CAD build for the part. Positions are in the model's coordinates, mm. A direction names the side the tool comes from. Round coordinates to 2 decimals unless told otherwise and drop trailing zeros. Order: outer loops, then holes, each group sorted by start corner. A loop starts at its lowest first (then second) coordinate and runs counter-clockwise, first axis right, second up. Notation, with made-up numbers: M -20.5,-5 L 15.5,-5 A21 cw 15.5,28 Z; hole C 81.5,-40 d2. An arc over 180 degrees is marked long. Answer as a JSON object with one key per item and string values.
```python
from build123d import *

# Parameters (mm, degrees)
EXTRUDE_3_DEPTH     = 1.7
SKETCH_4_R          = 0.81
EXTRUDE_4_DEPTH     = 3.7
SKETCH_5_W          = 79
SKETCH_5_H          = 14.47
EXTRUDE_5_DEPTH     = 5
SKETCH_6_W          = 79
SKETCH_6_H          = 31.63
EXTRUDE_6_DEPTH     = 5
FILLET_1_R          = 0.31
FILLET_2_R          = 0.5
FILLET_3_R          = 0.5
FILLET_5_R          = 0.5
SKETCH_8_W          = 40
SKETCH_8_H          = 31.63
EXTRUDE_7_DEPTH     = 5
FILLET_6_R          = 0.5
SKETCH_9_R          = 0.975
CUT_EXTRUDE_1_DEPTH = 5
FILLET_7_R          = 0.5


with BuildPart() as part:
    # 草图1 → 凸台-拉伸3 (new body)
    with BuildSketch(Plane.XY):
        with BuildLine():
            Line((0, 1.75), (55.5, 1.75))
            ThreePointArc((55.5, 1.75), (57.25, 0), (55.5, -1.75))
            Line((55.5, -1.75), (0, -1.75))
            ThreePointArc((0, -1.75), (-1.75, 0), (0, 1.75))
        make_face()
    extrude(amount=EXTRUDE_3_DEPTH)

    # 草图4 → 凸台-拉伸4 (add)
    with BuildSketch(Plane(origin=(0, 0, 0), x_dir=(-1, 0, 0), z_dir=(0, 0, -1))):
        Circle(SKETCH_4_R)
        with Locations((-55.5, 0)):
            Circle(SKETCH_4_R)
    extrude(amount=-EXTRUDE_4_DEPTH)

    # 草图5 → 凸台-拉伸5 (add)
    with BuildSketch(Plane(origin=(0, 0, 0), x_dir=(-1, 0, 0), z_dir=(0, 0, -1))):
        with Locations((-27.5, -1.005)):
            Rectangle(SKETCH_5_W, SKETCH_5_H)
    extrude(amount=EXTRUDE_5_DEPTH)

    # 草图6 → 凸台-拉伸6 (add)
    with BuildSketch(Plane(origin=(0, 6.23, 0), x_dir=(1, 0, 0), z_dir=(0, 1, 0))):
        with Locations((27.5, -10.815)):
            Rectangle(SKETCH_6_W, SKETCH_6_H)
    extrude(amount=EXTRUDE_6_DEPTH)

    # 圆角1
    fillet_1_edges = [part.edges().sort_by_distance(p)[0] for p in [
        (27.5, 6.23, 0),
    ]]
    fillet(fillet_1_edges, radius=FILLET_1_R)

    # 圆角2
    fillet_2_edges = [part.edges().sort_by_distance(p)[0] for p in [
        (67, -8.24, -2.5),
    ]]
    fillet(fillet_2_edges, radius=FILLET_2_R)

    # 圆角3
    fillet_3_edges = [part.edges().sort_by_distance(p)[0] for p in [
        (-12, -8.24, -2.5),
    ]]
    fillet(fillet_3_edges, radius=FILLET_3_R)

    # 圆角5
    fillet_5_edges = [part.edges().sort_by_distance(p)[0] for p in [
        (67, 11.23, 10.815),
    ]]
    fillet(fillet_5_edges, radius=FILLET_5_R)

    # 草图8 → 凸台-拉伸7 (add)
    with BuildSketch(Plane(origin=(0, -8.24, 0), x_dir=(-1, 0, 0), z_dir=(0, -1, 0))):
        with Locations((-35.5, -10.815)):
            Rectangle(SKETCH_8_W, SKETCH_8_H)
    extrude(amount=EXTRUDE_7_DEPTH)

    # 圆角6
    fillet_6_edges = [part.edges().sort_by_distance(p)[0] for p in [
        (67, 8.48, 26.63),
        (66.853553391, 11.083553391, 26.63),
        (2, -8.24, -5),
        (-11.853553391, -8.093553391, -5),
        (27.25, 11.23, -5),
        (66.853553391, 11.083553391, -5),
        (61, -8.24, -5),
        (66.853553391, -8.093553391, -5),
        (27.5, 6.23, 26.63),
        (-12, 8.73, 26.63),
        (27.25, 11.23, 26.63),
        (-12, 11.23, 10.815),
        (15.5, -8.24, 13.315),
        (15.5, -10.74, 26.63),
        (35.5, -8.24, 26.63),
        (55.5, -8.24, 13.315),
        (55.5, -10.74, 26.63),
        (55.5, -13.24, 10.815),
        (35.5, -13.24, 26.63),
        (15.5, -13.24, 10.815),
        (15.5, -10.74, -5),
        (-12, 1.745, -5),
        (55.5, -10.74, -5),
        (35.5, -13.24, -5),
        (67, 1.495, -5),
    ]]
    fillet(fillet_6_edges, radius=FILLET_6_R)

    # 草图9 → 切除-拉伸1 (cut)
    with BuildSketch(Plane.XY.offset(26.63)):
        with Locations((23.5, -10.74)):
            Circle(SKETCH_9_R)
        with Locations((47.5, -10.74)):
            Circle(SKETCH_9_R)
        with Locations((8, 8.73)):
            Circle(SKETCH_9_R)
        with Locations((47, 8.73)):
            Circle(SKETCH_9_R)
    extrude(amount=-CUT_EXTRUDE_1_DEPTH, mode=Mode.SUBTRACT)

    # 圆角7
    # the kernel refuses this fillet: 0.5 mm, written as the material it takes off along each edge
    with BuildSketch(Plane(origin=(-11.5, 6.73, 26.13), x_dir=(-1, 0, 0), z_dir=(0, -1, 0))) as fillet_7_piece_1_section:
        Polygon((0, 0), (FILLET_7_R * 1.02, 0), (FILLET_7_R * 1.02, -FILLET_7_R * 1.02), (0, -FILLET_7_R * 1.02), align=None)
    fillet_7_piece_1 = extrude(amount=FILLET_7_R * 1.02, mode=Mode.PRIVATE)
    fillet_7_piece_1 = fillet_7_piece_1 - Plane(origin=(-11.5, 6.73, 26.13), x_dir=(0.7071067811865475, 0, -0.7071067811865475), z_dir=(0, -1, 0)) * Sphere(FILLET_7_R, mode=Mode.PRIVATE)
    add(fillet_7_piece_1, mode=Mode.SUBTRACT)
    with BuildSketch(Plane(origin=(66.5, 6.73, 26.13), x_dir=(0, -1, 0), z_dir=(1, 0, 0))) as fillet_7_piece_2_section:
        Polygon((0, 0), (FILLET_7_R * 1.02, 0), (FILLET_7_R * 1.02, -FILLET_7_R * 1.02), (0, -FILLET_7_R * 1.02), align=None)
    fillet_7_piece_2 = extrude(amount=FILLET_7_R * 1.02, mode=Mode.PRIVATE)
    fillet_7_piece_2 = fillet_7_piece_2 - Plane(origin=(66.5, 6.73, 26.13), x_dir=(0, 0.7071067811865475, -0.7071067811865475), z_dir=(1, 0, 0)) * Sphere(FILLET_7_R, mode=Mode.PRIVATE)
    add(fillet_7_piece_2, mode=Mode.SUBTRACT)
    with BuildSketch(Plane(origin=(-12, 5.92, 0), x_dir=(1, 0, 0), z_dir=(0, -1, 0))) as fillet_7_piece_3:
        with BuildLine():
            CenterArc((FILLET_7_R, -FILLET_7_R), FILLET_7_R, 90, 90)
            Line((0, -FILLET_7_R), (0, 0))
            Line((0, 0), (FILLET_7_R, 0))
        make_face()
    extrude(amount=13.66, mode=Mode.SUBTRACT)
    with BuildSketch(Plane(origin=(67, -7.74, 0), x_dir=(0, 0, -1), z_dir=(0, 1, 0))) as fillet_7_piece_4:
        with BuildLine():
            CenterArc((FILLET_7_R, FILLET_7_R), FILLET_7_R, 180, 90)
            Line((0, FILLET_7_R), (0, 0))
            Line((0, 0), (FILLET_7_R, 0))
        make_face()
    extrude(amount=13.66, mode=Mode.SUBTRACT)
    with BuildSketch(Plane(origin=(-12, 6.23, 26.13), x_dir=(1, 0, 0), z_dir=(0, 0, -1))) as fillet_7_piece_5:
        with BuildLine():
            CenterArc((FILLET_7_R, -FILLET_7_R), FILLET_7_R, 90, 90)
            Line((0, -FILLET_7_R), (0, 0))
            Line((0, 0), (FILLET_7_R, 0))
        make_face()
    extrude(amount=25.82, mode=Mode.SUBTRACT)
    with BuildSketch(Plane(origin=(-12, 5.92, 0.31), x_dir=(0, 0, -1), z_dir=(0, -1, 0))) as fillet_7_piece_6:
        with BuildLine():
            CenterArc((0.31 + FILLET_7_R, FILLET_7_R), FILLET_7_R, 180, 90)
            Line((0.31 + FILLET_7_R, 0), (0.31, 0))
            Line((0.31, 0), (0.31, FILLET_7_R))
        make_face()
    revolve(axis=Axis((-12, 5.92, 0.31), (1, 0, 0)), revolution_arc=90, mode=Mode.SUBTRACT)
    with BuildSketch(Plane(origin=(67, 5.92, 0.31), x_dir=(0, 0, -1), z_dir=(0, -1, 0))) as fillet_7_piece_7:
        with BuildLine():
            CenterArc((0.31 + FILLET_7_R, -FILLET_7_R), FILLET_7_R, 90, 90)
            Line((0.31, -FILLET_7_R), (0.31, 0))
            Line((0.31, 0), (0.31 + FILLET_7_R, 0))
        make_face()
    revolve(axis=Axis((67, 5.92, 0.31), (1, 0, 0)), revolution_arc=90, mode=Mode.SUBTRACT)
    with BuildSketch(Plane(origin=(55.5, -8.24, 0), x_dir=(0, 1, 0), z_dir=(1, 0, 0))) as fillet_7_piece_8:
        with BuildLine():
            CenterArc((FILLET_7_R, -FILLET_7_R), FILLET_7_R, 90, 90)
            Line((0, -FILLET_7_R), (0, 0))
            Line((0, 0), (FILLET_7_R, 0))
        make_face()
    extrude(amount=11, mode=Mode.SUBTRACT)
    with BuildSketch(Plane(origin=(66.5, -7.74, 0), x_dir=(1, 0, 0), z_dir=(0, 1, 0))) as fillet_7_piece_9:
        with BuildLine():
            CenterArc((0.5 - FILLET_7_R, FILLET_7_R), FILLET_7_R, 270, 90)
            Line((0.5 - FILLET_7_R, 0), (0.5, 0))
            Line((0.5, 0), (0.5, FILLET_7_R))
        make_face()
    revolve(axis=Axis((66.5, -7.74, 0), (0, 0, -1)), revolution_arc=90, mode=Mode.SUBTRACT)
    with BuildSketch(Plane(origin=(-11.5, -7.74, 0), x_dir=(0, -1, 0), z_dir=(1, 0, 0))) as fillet_7_piece_10:
        with BuildLine():
            CenterArc((0.5 - FILLET_7_R, FILLET_7_R), FILLET_7_R, 270, 90)
            Line((0.5, FILLET_7_R), (0.5, 0))
            Line((0.5, 0), (0.5 - FILLET_7_R, 0))
        make_face()
    revolve(axis=Axis((-11.5, -7.74, 0), (0, 0, -1)), revolution_arc=90, mode=Mode.SUBTRACT)
    with BuildSketch(Plane(origin=(-11.5, -8.24, 0), x_dir=(0, 1, 0), z_dir=(1, 0, 0))) as fillet_7_piece_11:
        with BuildLine():
            CenterArc((FILLET_7_R, -FILLET_7_R), FILLET_7_R, 90, 90)
            Line((0, -FILLET_7_R), (0, 0))
            Line((0, 0), (FILLET_7_R, 0))
        make_face()
    extrude(amount=27, mode=Mode.SUBTRACT)
    with BuildSketch(Plane(origin=(67, 6.23, 0.31), x_dir=(0, 1, 0), z_dir=(0, 0, 1))) as fillet_7_piece_12:
        with BuildLine():
            CenterArc((FILLET_7_R, FILLET_7_R), FILLET_7_R, 180, 90)
            Line((0, FILLET_7_R), (0, 0))
            Line((0, 0), (FILLET_7_R, 0))
        make_face()
    extrude(amount=25.82, mode=Mode.SUBTRACT)


solid = part.part
```
Item 1: Two-plate mould, pull along X, no slides. Class faces 6 (the flat face through (55.5, -11, 11)), 7 (the cylindrical face through (0.18, -0.79, 2.69)), 8 (the flat face through (36, -11, 26.63)): released by +X, released by -X, zero draft, split by the parting line, or undercut.
Worked answers:
{"face 6": "released by +X", "face 7": "undercut", "face 8": "zero draft"}
Item 2: Saw through at D-D on x = 23.5. List the corners of the cut face in (y, z) (3 decimals), and give its area (3 significant figures).
Worked answers:
{"outline": "M -13.24,-4.5 A0.5 ccw -12.74,-5 L 10.73,-5 A0.5 ccw 11.23,-4.5 L 11.23,26.13 A0.5 ccw 10.73,26.63 L 6.73,26.63 A0.5 ccw 6.23,26.13 L 6.23,0.31 A0.31 cw 5.92,0 L 1.75,0 L 1.75,1.7 L -1.75,1.7 L -1.75,0 L -8.24,0 L -8.24,26.13 A0.5 ccw -8.74,26.63 L -9.765,26.63 L -9.765,21.63 L -11.715,21.63 L -11.715,26.63 L -12.74,26.63 A0.5 ccw -13.24,26.13 Z", "area": "385 mm2"}
Item 3: Saw through at A-A on z = 24. List the corners of the cut face in (x, y) (3 decimals), and give its area (3 significant figures).
Worked answers:
{"outline": "M -12,6.73 A0.5 ccw -11.5,6.23 L 66.5,6.23 A0.5 ccw 67,6.73 L 67,10.73 A0.5 ccw 66.5,11.23 L -11.5,11.23 A0.5 ccw -12,10.73 Z; M 15.5,-12.74 A0.5 ccw 16,-13.24 L 55,-13.24 A0.5 ccw 55.5,-12.74 L 55.5,-8.74 A0.5 ccw 55,-8.24 L 16,-8.24 A0.5 ccw 15.5,-8.74 Z; hole C 8,8.73 d1.95; hole C 23.5,-10.74 d1.95; hole C 47,8.73 d1.95; hole C 47.5,-10.74 d1.95", "area": "583 mm2"}
Item 4: Saw through at B-B on z = 18. List the corners of the cut face in (x, y), and give its area (3 significant figures).
Worked answers:
{"outline": "M -12,6.73 A0.5 ccw -11.5,6.23 L 66.5,6.23 A0.5 ccw 67,6.73 L 67,10.73 A0.5 ccw 66.5,11.23 L -11.5,11.23 A0.5 ccw -12,10.73 Z; M 15.5,-12.74 A0.5 ccw 16,-13.24 L 55,-13.24 A0.5 ccw 55.5,-12.74 L 55.5,-8.74 A0.5 ccw 55,-8.24 L 16,-8.24 A0.5 ccw 15.5,-8.74 Z", "area": "595 mm2"}
Item 5: Wall check: line 1 along Y through (x, z) = (23.5, 24.1) (3 decimals); line 2 along Y through (x, z) = (55, 10); line 3 along Y through (x, z) = (47, 25) (3 decimals). Give the ranges that are in metal, low to high. Write a range as [from, to].
Worked answers:
{"line 1": "y = [-13.24, -11.715], [-9.765, -8.24], [6.23, 11.23]", "line 2": "y = [-13.24, -8.24], [6.23, 11.23]", "line 3": "y = [-13.24, -11.577], [-9.903, -8.24], [6.23, 7.755], [9.705, 11.23]"}
Item 6: 3-axis set-ups, long thin cutter, end or side, ignore diameter. For faces 1 (the cylindrical face through (24.024, -9.918, 24.165)), 2 (the flat face through (27, 6.23, 13)), 3 (the flat face through (61, -8.24, -2)), 4 (the cylindrical face through (57.25, 0.04, 0.84)), 5 (the flat face through (2, -8.24, -2)): which of +Z, -Z, +X, -X, +Y, -Y reach the whole face in a straight line?
Worked answers:
{"face 1": "+Z", "face 2": "+Z, +X, -X", "face 3": "+Z, -Z, +X, -Y", "face 4": "+Z, +X", "face 5": "+Z, -Z, -X, -Y"}
Item 7: Saw through at C-C on y = -3. List the corners of the cut face in (x, z).
Worked answers:
{"outline": "M -12,-4.5 A0.5 ccw -11.5,-5 L 66.5,-5 A0.5 ccw 67,-4.5 L 67,-0.5 A0.5 ccw 66.5,0 L -11.5,0 A0.5 ccw -12,-0.5 Z"}
Item 8: Drop flat-ended pins along their axis: pin 1 Ø5 at (x, y) = (7.5, 1.5) entering from +Z; pin 2 Ø3 at (x, z) = (61.5, -3) entering from -Y; pin 3 Ø0.8 at (x, y) = (55, -0.5) entering from +Z. Give the stop position or say it passes through.
Worked answers:
{"pin 1": "stops at z = 1.7", "pin 2": "stops at y = -8.24", "pin 3": "stops at z = 3.7"}
